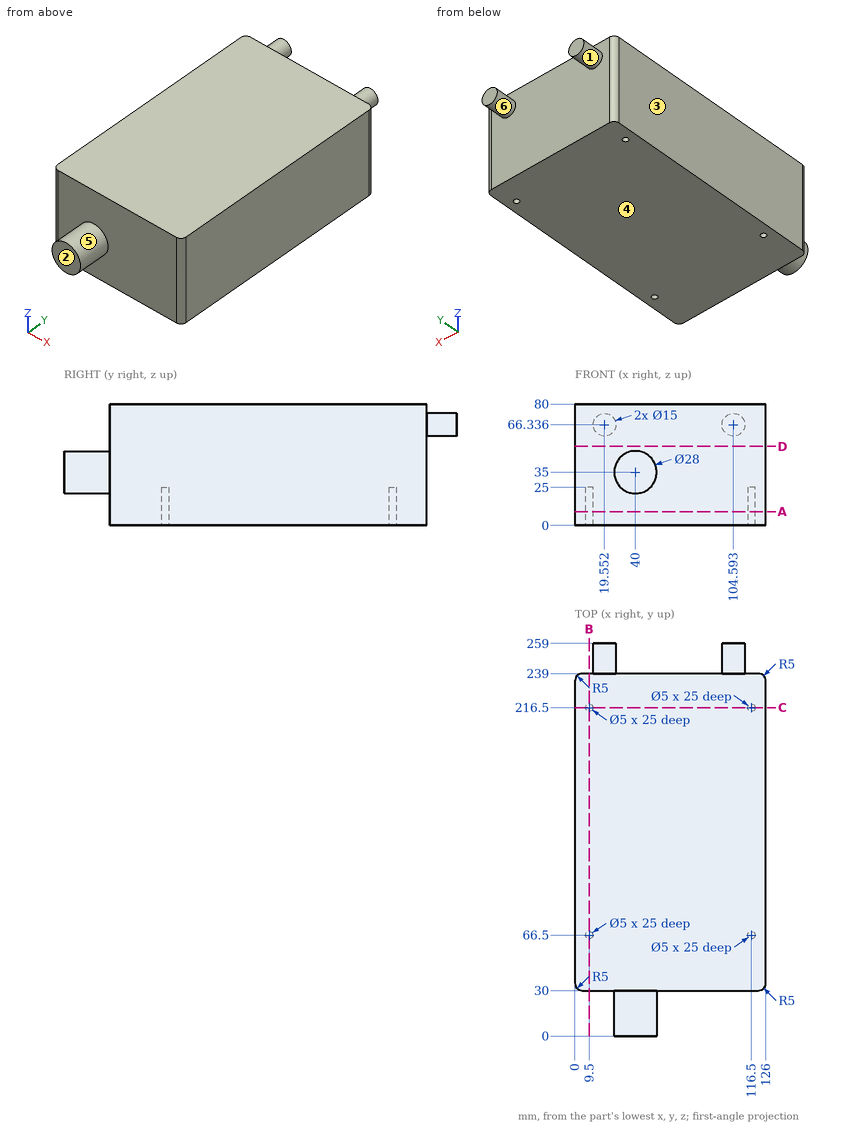
The drawing under review shows one solid part. Ordinate dimensions are in mm from its lowest x, y, z. A direction names the side the tool comes from. Round coordinates to 2 decimals unless told otherwise and drop trailing zeros. Loops run counter-clockwise (first coordinate to the right, second up) from the corner with the lowest first, then second, coordinate; pieces in that order, holes last. Notation, with made-up numbers: (20, -38.5) - (42, -38.5) arc R13 cw to (42, -25.5) - close; hole circle Ø5 at (15, 66.25). An arc over 180 degrees is marked (long way). One line per question, with ' | ' between items.
Q1. Tool access review of the marked faces 4, 5 and 6: name each direction out of +Z, -Z, +X, -X, +Y, -Y from which nothing blocks a thin tool from reaching the whole face with its end or side.
Taken from the geometry:
face 4: -Z, +X, -X, +Y, -Y | face 5: -Y | face 6: +Y
Q2. Take a section at B-B (x = 9.5). Give the boundary of the cut face in (y, z), and give its area (3 significant figures).
Taken from the geometry:
outline: (30, 0) - (64, 0) - (64, 25) - (69, 25) - (69, 0) - (214, 0) - (214, 25) - (219, 25) - (219, 0) - (239, 0) - (239, 80) - (30, 80) - close | area: 16,500 mm²
Q3. Take a section at A-A (z = 9). Give the boundary of the cut face in (x, y), and give its area (3 significant figures).
Taken from the geometry:
outline: (0, 35) arc R5 ccw to (5, 30) - (121, 30) arc R5 ccw to (126, 35) - (126, 234) arc R5 ccw to (121, 239) - (5, 239) arc R5 ccw to (0, 234) - close; hole circle Ø5 at (9.5, 66.5); hole circle Ø5 at (9.5, 216.5); hole circle Ø5 at (116.5, 66.5); hole circle Ø5 at (116.5, 216.5) | area: 26,200 mm²
Q4. Take a section at D-D (z = 52). Give the boundary of the cut face in (x, y), and give its area (3 significant figures).
Taken from the geometry:
outline: (0, 35) arc R5 ccw to (5, 30) - (121, 30) arc R5 ccw to (126, 35) - (126, 234) arc R5 ccw to (121, 239) - (5, 239) arc R5 ccw to (0, 234) - close | area: 26,300 mm²
Q5. Take a section at C-C (y = 216.5). Give the boundary of the cut face in (x, z), and give its area (3 significant figures).
Taken from the geometry:
outline: (0, 0) - (7, 0) - (7, 25) - (12, 25) - (12, 0) - (114, 0) - (114, 25) - (119, 25) - (119, 0) - (126, 0) - (126, 80) - (0, 80) - close | area: 9,830 mm²
Q6. For line 1 along Y through (x, z) = (116, 10); line 2 along X through (y, z) = (216, 17); line 3 along X through (y, z) = (216.5, 7.5), list the stretches that pass through material, from the lowest coordinate up. Write a range as [from, to].
Taken from the geometry:
line 1: y = [30, 64.05], [68.95, 214.05], [218.95, 239] | line 2: x = [0, 7.05], [11.95, 114.05], [118.95, 126] | line 3: x = [0, 7], [12, 114], [119, 126]
Q7. For pin 1 (4 mm diameter, centred on x = 116.5, y = 66.5, fed in from -Z); pin 2 (1 mm diameter, centred on x = 42, z = 54, fed in from +Y), all flat-tipped, find the tip position at first contact; note any pin that passes through.
Taken from the geometry:
pin 1: stops at z = 25 | pin 2: stops at y = 239
Q8. The part is to be moulded in two halves that separate along X. For the marked faces 1, 2 and 3, say which applies: released by +X, released by -X, zero draft, split by the parting line, or undercut.
Taken from the geometry:
face 1: undercut | face 2: zero draft | face 3: released by -X
